Source: CAD feature listing. Evaluate the final solid. Frame: model axes, mm. Round coordinates to 2 decimals unless told otherwise and drop trailing zeros. Order: outer loops, then holes, each group sorted by start corner. A loop starts at its lowest first (then second) coordinate and runs counter-clockwise, first axis right, second up. Notation, with made-up numbers: (85.5, 87) -> (126.5, 87) arc R18 ccw to (126.5, 92) -> close; hole circle Ø3 at (16.5, 82.5). An arc over 180 degrees is marked (long way). Write item = value, one per line. Start each with the question number.
(1) Contact query for flat-ended pins moving along their axis: pin 1 Ø7.5 at (x, y) = (-52, 143.5) entering from +Z; pin 2 Ø3 at (y, z) = (12.5, 3) entering from -X; pin 3 Ø3 at (y, z) = (38, 4.5) entering from +X. Output: stop coordinate, or through.
(2) Cut plane C-C on z = 8.5. Return the cut outline in (x, y).
(3) Cut plane B-B on y = -41. Return the cut outline in (x, z), then the cut area to 3 significant figures.
(4) Ray query, line 1 (X direction, y = -125, z = 5); line 2 (Z direction, x = 75, y = -73.5). Return the intervals inside material, ascending.
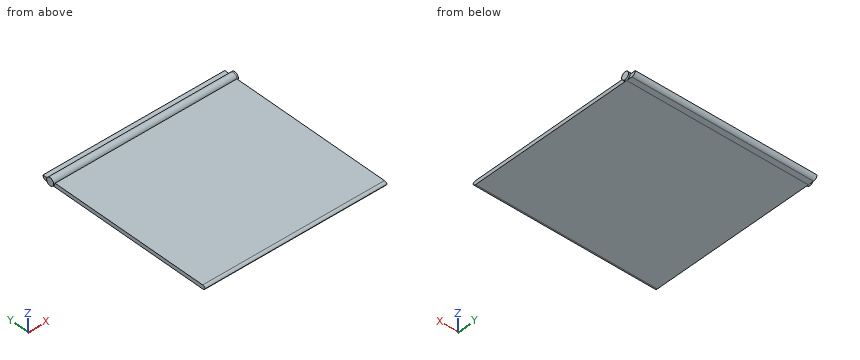
from build123d import *

# Parameters (mm, degrees)
F0_W          = 304.8
F0_H          = 298.45
F1_DEPTH      = 6.35
F2_R          = 6.34999
F3_R          = 6.35
F4_DEPTH      = 2.54
F4_DEPTH_BACK = 307.34
F5_T1_DEPTH   = 330.2


# Not quite as in the source:
# - a fillet or chamfer that OpenCascade refuses, or shapes differently, is made with other operations: its cross-section is extruded or revolved along the edge and cut away or added
# - a fillet or chamfer is up to 0.001 mm smaller than in the source, because OpenCascade refuses the exact size


with BuildPart() as f1:
    # F0 (on Top) → F1 (new body)
    with BuildSketch(Plane.XY):
        Rectangle(F0_W, F0_H)
    extrude(amount=F1_DEPTH)

    # F2 (radius 6.35 in the source; OpenCascade refuses exactly that, so slightly less here)
    f2_edges = [f1.edges().sort_by_distance(p)[0] for p in [
        (0, 149.225, 0),
    ]]
    fillet(f2_edges, radius=F2_R)

    # F3 (on face) → F4 (join, two sides)
    with BuildSketch(Plane.YZ.offset(152.4)) as f4_sk:
        with Locations((133.35, 6.35)):
            Circle(F3_R)
    extrude(amount=F4_DEPTH)
    extrude(f4_sk.sketch, amount=-F4_DEPTH_BACK)

    # F5: fillet of radius 5.08 on 2 edges, made by hand

    # F5_s2 → F5_t1 (cut)
    with BuildSketch(Plane.YZ.offset(-165.1)):
        with BuildLine():
            ThreePointArc((-144.145, 0), (-147.7371024484, 1.4878975516), (-149.225, 5.08))
            Line((-149.225, 5.08), (-149.225, 0))
            Line((-149.225, 0), (-144.145, 0))
        make_face()
        with BuildLine():
            ThreePointArc((-144.145, 6.35), (-147.7371024484, 4.8621024484), (-149.225, 1.27))
            Line((-149.225, 1.27), (-149.225, 6.35))
            Line((-149.225, 6.35), (-144.145, 6.35))
        make_face()
    extrude(amount=F5_T1_DEPTH, mode=Mode.SUBTRACT)


solid = f1.part
Evaluation:
q1.pin_1 = 6.35
q1.pin_2 = -152.4
q1.pin_3 = 152.4
q2.outline = (-154.94, 127.38) -> (154.94, 127.38) -> (154.94, 139.32) -> (-154.94, 139.32) -> close
q3.outline = (-152.4, 0) -> (152.4, 0) -> (152.4, 6.35) -> (-152.4, 6.35) -> close
q3.area = 1,940 mm^2
q4.line_1 = -152.4 to 152.4
q4.line_2 = 0 to 6.35
